Geometry check sheet. Reference: the model listing, model coordinates, mm. A direction names the side the tool comes from. Round coordinates to 2 decimals unless told otherwise and drop trailing zeros. Write each loop counter-clockwise with the first axis right and the second up, starting at its lowest first coordinate (ties: lowest second). Pieces come first, ordered by that corner, then holes. Notation, with made-up numbers: (6.5, 78.5) - (62.5, 78.5) arc R9 cw to (62.5, 84.5) - close; hole circle Ø6 at (16.25, 79.5). An arc over 180 degrees is marked (long way). Return JSON: item names as keys, results as strings. Group by question number.
from build123d import *

# Parameters (mm, degrees)
F1_DEPTH = 6
F3_DEPTH = 3
F3_TAPER = 10
F4_SIZE  = 1
F5_W     = 2.5
F5_H     = 2.5
F6_DEPTH = 2
F7_R     = 2.5
F8_DEPTH = 3


with BuildPart() as f1:
    # F0 (on Top) → F1 (new body)
    with BuildSketch(Plane.XY):
        Polygon((0, 20), (0, 0), (20, 0), (36.3692647093, 18.5151209051), (36.3692647093, 38.5151209051), (16.3692647093, 38.5151209051), align=None)
    extrude(amount=F1_DEPTH)

    # F2 (on face) → F3 (cut)
    with BuildSketch(Plane.XY.offset(6)):
        Polygon((2, 19.2426673516), (2, 2), (19.0986453142, 2), (34.3692647093, 19.2724535535), (34.3692647093, 36.5151209051), (17.2706193952, 36.5151209051), align=None)
    extrude(amount=-F3_DEPTH, taper=F3_TAPER, mode=Mode.SUBTRACT)

    # F4
    f4_edges = [f1.edges().sort_by_distance(p)[0] for p in [
        (0, 0, 3),
        (36.369265, 38.515121, 3),
    ]]
    chamfer(f4_edges, length=F4_SIZE)

    # F5 (on face) → F6 (cut)
    with BuildSketch(Plane.XY.offset(6)):
        with Locations((1.25, 1.25)):
            Rectangle(F5_W, F5_H)
        with Locations((35.1192647093, 37.2651209051)):
            Rectangle(F5_W, F5_H)
    extrude(amount=-F6_DEPTH, mode=Mode.SUBTRACT)

    # F7 (on face) → F8 (cut, through all)
    with BuildSketch(Plane.XY.offset(3)):
        with Locations((12.5289809421, 12.5289809421)):
            Circle(F7_R)
        with Locations((23.8402837672, 25.9861399629)):
            Circle(F7_R)
    extrude(amount=-F8_DEPTH, mode=Mode.SUBTRACT)


solid = f1.part
1. Material ranges on line 1 along Z through (x, y) = (24.5, 15.5); line 2 along X through (y, z) = (32, 5); line 3 along Y through (x, z) = (33.5, 3.25), recorded low to high.
2. Section check A-A (z = 0.5). Enter the section's corners in (x, y), and give its area (3 significant figures).
3. Mould release check, pull along Y, two halves, no side actions. Record for faces 1 (the face through (8.3, 29.39, 2.96)), 2 (the face through (10.545, 11.008, 1.521)), 3 (the face through (28.07, 9.13, 2.96)): pulls with the +Y half, pulls with the -Y half, needs draft (parallel to the pull), parting line crosses it, or undercut.
4. Tool access check on faces 4 (the face through (33.869, 37, 5)), 5 (the face through (18, 19, 3)), 6 (the face through (2.5, 1, 5)). Record the directions out of +Z, -Z, +X, -X, +Y, -Y that give a thin tool (end or side, any length) a straight path to the whole face; none if there is none.
5. Depth check by flat-ended pin: pin 1 Ø1.6 at (x, z) = (35, 5) entering from +Y; pin 2 Ø1 at (x, y) = (15, 6) entering from +Z; pin 3 Ø2 at (y, z) = (1.5, 4.5) entering from -X; pin 4 Ø0.6 at (y, z) = (37.5, 5) entering from +X. Enter the tip coordinate at first touch or a pass-through.
Result sheet:
{
 "1": {"line 1": "z = 0 to 3", "line 2": "x = 10.61 to 13.51, 34.19 to 36.37", "line 3": "y = 15.27 to 19.02, 36.03 to 38.52"},
 "2": {"outline": "(0, 1) - (1, 0) - (20, 0) - (36.37, 18.52) - (36.37, 37.52) - (35.37, 38.52) - (16.37, 38.52) - (0, 20) - close; hole circle Ø5 at (12.53, 12.53); hole circle Ø5 at (23.84, 25.99)", "area": "1,060 mm²"},
 "3": {"face 1": "pulls with the +Y half", "face 2": "undercut", "face 3": "pulls with the -Y half"},
 "4": {"face 4": "+Z, +X, +Y", "face 5": "+Z", "face 6": "+Z, -X, -Y"},
 "5": {"pin 1": "stops at y = 36.02", "pin 2": "stops at z = 3", "pin 3": "stops at x = 0", "pin 4": "stops at x = 33.87"}
}
